Input: part model. Units: mm. Frame: model coordinates. A direction names the side the tool comes from. Give positions to 0.01 mm unless a question says otherwise; leave off trailing zeros. Loops run counter-clockwise (first coordinate to the right, second up) from the corner with the lowest first, then second, coordinate; pieces in that order, holes last. Notation, with made-up numbers: (6.25, 0.25) -> (44.25, 0.25) arc R23 ccw to (44.25, 19.25) -> close; hole circle Ø1 at (88.5, 20). An arc over 180 degrees is marked (long way). One line per question, with ' | ' between items.
from build123d import *

# Parameters (mm, degrees)
SKETCH1_W           = 76.2
SKETCH1_H           = 50.8
SKETCH1_R           = 6.35
BOSS_EXTRUDE1_DEPTH = 33.02
SKETCH2_W           = 27.94
SKETCH2_H           = 60.96
CUT_EXTRUDE1_DEPTH  = 87.844230666
SKETCH3_R           = 6.35
CUT_EXTRUDE2_DEPTH  = 70.792248853
FILLET1_R           = 2.54


with BuildPart() as part:
    # Sketch1 → Boss-Extrude1 (new body)
    with BuildSketch(Plane.XY):
        Rectangle(SKETCH1_W, SKETCH1_H)
        with Locations((0, -12.7)):
            Circle(SKETCH1_R, mode=Mode.SUBTRACT)
    extrude(amount=BOSS_EXTRUDE1_DEPTH)

    # Sketch2 → Cut-Extrude1 (cut, through all)
    with BuildSketch(Plane(origin=(38.1, 0, 0), x_dir=(0, 0, -1), z_dir=(1, 0, 0))):
        with Locations((-16.51, -7.62)):
            Rectangle(SKETCH2_W, SKETCH2_H)
    extrude(amount=-CUT_EXTRUDE1_DEPTH, mode=Mode.SUBTRACT)

    # Sketch3 → Cut-Extrude2 (cut, through all)
    with BuildSketch(Plane.XZ.offset(-22.86)):
        with Locations((0, 16.51)):
            Circle(SKETCH3_R)
    extrude(amount=-CUT_EXTRUDE2_DEPTH, mode=Mode.SUBTRACT)

    # Fillet1
    fillet1_edges = [part.edges().sort_by_distance(p)[0] for p in [
        (0, 25.4, 0),
        (0, 25.4, 33.02),
    ]]
    fillet(fillet1_edges, radius=FILLET1_R)


solid = part.part
1. Section query A-A (x = 0). Output: boundary loops of the cut face in (y, z), then the cut area to 3 significant figures.
Determined:
outline: (-25.4, 0) -> (-19.05, 0) -> (-19.05, 2.54) -> (-25.4, 2.54) -> close; (-25.4, 30.48) -> (-19.05, 30.48) -> (-19.05, 33.02) -> (-25.4, 33.02) -> close; (-6.35, 0) -> (22.86, 0) arc R2.54 ccw to (25.4, 2.54) -> (25.4, 10.16) -> (22.86, 10.16) -> (22.86, 2.54) -> (-6.35, 2.54) -> close; (-6.35, 30.48) -> (22.86, 30.48) -> (22.86, 22.86) -> (25.4, 22.86) -> (25.4, 30.48) arc R2.54 ccw to (22.86, 33.02) -> (-6.35, 33.02) -> close | area: 229 mm2
2. Section query C-C (y = -12.7). Output: boundary loops of the cut face in (x, z), then the cut area to 3 significant figures.
Determined:
outline: (-38.1, 0) -> (-6.35, 0) -> (-6.35, 2.54) -> (-38.1, 2.54) -> close; (-38.1, 30.48) -> (-6.35, 30.48) -> (-6.35, 33.02) -> (-38.1, 33.02) -> close; (6.35, 0) -> (38.1, 0) -> (38.1, 2.54) -> (6.35, 2.54) -> close; (6.35, 30.48) -> (38.1, 30.48) -> (38.1, 33.02) -> (6.35, 33.02) -> close | area: 323 mm2
3. Pull-direction query (Z, two-part tool) for faces 1 (the cylindrical face through (0.533, 24.676, 32.256)), 2 (the flat face through (1, -2, 30.48)), 3 (the flat face through (-1, 25.4, 10)); classes: pulls with the +Z half, pulls with the -Z half, needs draft (parallel to the pull), parting line crosses it, or undercut.
Determined:
face 1: pulls with the +Z half | face 2: undercut | face 3: needs draft
4. Section query D-D (y = 18.5). Output: boundary loops of the cut face in (x, z), then the cut area to 3 significant figures.
Determined:
outline: (-38.1, 0) -> (38.1, 0) -> (38.1, 2.54) -> (-38.1, 2.54) -> close; (-38.1, 30.48) -> (38.1, 30.48) -> (38.1, 33.02) -> (-38.1, 33.02) -> close | area: 387 mm2
5. Section query B-B (z = 16.51). Output: boundary loops of the cut face in (x, y).
Determined:
outline: (-38.1, 22.86) -> (-6.35, 22.86) -> (-6.35, 25.4) -> (-38.1, 25.4) -> close; (6.35, 22.86) -> (38.1, 22.86) -> (38.1, 25.4) -> (6.35, 25.4) -> close
6. Pin query (flat end, axial travel): P1, Ø4, axis at y = -10.5, z = 29, coming from the -X side; P2, Ø1.5, axis at x = -4.5, z = 25.5, coming from the -Y side; P3, Ø7.5, axis at x = 0, y = -12.7, coming from the +Z side. Return the tip coordinate at first contact, or that it passes through.
Determined:
P1: stops at x = -38.1 | P2: stops at y = 22.86 | P3: passes through
7. Ray query, line 1 along X through (y, z) = (-12.7, 0.75); line 2 along Z through (x, y) = (-19.5, 18); line 3 along Z through (x, y) = (0, 24.85). Return the intervals inside material, ascending. Write a range as from..to.
Determined:
line 1: x = -38.1..-6.35, 6.35..38.1 | line 2: z = 0..2.54, 30.48..33.02 | line 3: z = 0.96..10.16, 22.86..32.06
8. Reachability of faces 4 (the flat face through (1, -2, 2.54)), 5 (the cylindrical face through (-1.38, -18.9, 31.73)) from +Z, -Z, +X, -X, +Y, -Y: full face, straight path, thin tool, end or side. Return the list, or none.
Determined:
face 4: +X, -X, -Y | face 5: +Z, -Z
